Read the model definition and answer for the solid it produces. Units are mm, in the model's axes. A direction names the side the tool comes from. Coordinates: 2 decimals unless noted, no trailing zeros. Loops run counter-clockwise (first coordinate to the right, second up) from the corner with the lowest first, then second, coordinate; pieces in that order, holes last. Notation, with made-up numbers: (14.25, 39.5) - (35.25, 39.5) arc R30 ccw to (35.25, 62.5) - close; hole circle Ø10 at (86.5, 53). An arc over 180 degrees is marked (long way). Use one line per item in the form item = value. Start each with the question number.
1) A cutting plane is placed at A-A (y = 368.3). Give the vertices of the cut face in (x, z) (3 decimals), and give its area (3 significant figures).
2) A cutting plane is placed at B-B (z = -4.5). Give the vertices of the cut face in (x, y) (3 decimals), and give its area (3 significant figures).
3) Which of the six approach directions +Z, -Z, +X, -X, +Y, -Y give full straight-line access (tool end or side, diameter ignored) to faces 1 (the face through (-9.525, 363, 0)), 2 (the face through (-0.279, 730.244, -11.135))?
4) The mould has two halves that part along Y. Classify faces 3 (the face through (-0.279, 730.244, 11.09)), 4 (the face through (9.525, 363, 0)), 5 (the face through (-11, 0, 0)): released by +Y, released by -Y, zero draft, split by the parting line, or undercut.
5) A cutting plane is placed at C-C (y = 555.5). Give the vertices of the cut face in (x, z) (3 decimals).
6) Consider line 1 (Y direction, x = 0, z = -10.25); line 2 (Z direction, x = 3.75, y = 134) (3 decimals); line 3 (X direction, y = 12.7, z = -11.3). Determine where each line is inside the solid, lowest interval first.
7) This flat-tipped pin is pushed along its axis until it touches: P1, Ø14.5, axis at x = 0, y = 368.3, coming from the +Z side. Where does it stop, or does it pass through?
Autodesk Inventor part; units mm, degrees
ref_plane "YZ Plane" through (0, 0, 0) normal (1, 0, 0) x (0, 1, 0)
ref_plane "XZ Plane" through (0, 0, 0) normal (0, 1, 0) x (-1, 0, 0)
ref_plane "XY Plane" through (0, 0, 0) normal (0, 0, 1) x (1, 0, 0)
sketch "Sketch1" plane through (0, 0, 0) normal (0, 1, 0) x (-1, 0, 0)
  line L0 (12.7, 12.7) -> (-12.7, 12.7)
  line L1 (-12.7, 12.7) -> (-12.7, -12.7)
  line L2 (-12.7, -12.7) -> (12.7, -12.7)
  line L3 (12.7, -12.7) -> (12.7, 12.7)
  line L4 (-9.525, 9.525) -> (9.525, 9.525)
  line L5 (9.525, 9.525) -> (9.525, -9.525)
  line L6 (9.525, -9.525) -> (-9.525, -9.525)
  line L7 (-9.525, -9.525) -> (-9.525, 9.525)
  point P0 (0, 0)
  point P1 (12.7, 0)
  point P2 (0, -12.7)
  dimension "d0" = 25.4
  dimension "d1" = 25.4
  dimension "d2" = 3.175
extrude "Extrusion1" add sketch "Sketch1" along normal blind 736.6
sketch "Sketch2" plane through (-12.7, 0, 12.7) normal (0, 0, 1) x (1, 0, 0)
  line L0 (0, 736.6) -> (25.4, 736.6)
  line L1 (0, 0) -> (25.4, 0)
  point P0 (12.7, 0)
  point P1 (12.7, 12.7)
  point P2 (12.7, 723.9)
  point P3 (12.7, 368.3)
  dimension "d5" = 12.7
  dimension "d6" = 12.7
  dimension "d7" = 368.3
hole "Hole1" at (0, 12.7, 12.7) at (0, 723.9, 12.7) at (0, 368.3, 12.7) direction (0, 0, -1) diameter 12.7 end through all
sketch "Sketch3" plane through (-12.7, 0, 12.7) normal (0, 0, 1) x (1, 0, 0)
  line L0 (21.6869, 114.0639) -> (21.6869, 96.9638) construction
  line L1 (21.6869, 96.9638) -> (5.8083, 96.9638) construction
  line L2 (5.8083, 96.9638) -> (5.8083, 114.0639) construction
  line L3 (5.8083, 114.0639) -> (21.6869, 114.0639) construction
  point P0 (12.7, 0)
sketch "Sketch4" plane through (12.7, 0, -12.7) normal (0, 0, -1) x (-1, 0, 0)
  circle A0 centre (12.7, 635.3302) radius 3.175
  line L0 (0, 736.6) -> (25.4, 736.6)
  point P0 (12.7, 0)
  dimension "d15" = 101.2698
  dimension "d16" = 6.35
extrude "Extrusion2" cut sketch "Sketch4" against normal through all
equation "\"d0\" = Tube_size"
equation "\"d1\" = Tube_size"
equation "\"d2\" = Wall_Thickness"
equation "\"d3\" = Bar3_1_Length"
equation "\"d8\" = Pin_Size"
equation "\"Bar1_1_Length\" = 736.6"
equation "\"Tube_size_1\" = 25.4"
equation "\"Wall_Thickness_1\" = 3.175"
equation "\"Lower_Pivit_Offset_FromEdge\" = 12.7"
equation "\"Uper_Pivit_Offset_FromEdge\" = 12.7"
equation "\"Bar1_1_Center_Pivit_Offset_FromEdge\" = 368.3"
equation "\"Bar1_2_Length\" = 736.6"
equation "\"Bar2_1_Length\" = 736.6"
equation "\"Bar2_2_Length\" = 736.6"
equation "\"Bar3_1_Length\" = 736.6"
equation "\"Bar3_2_Length\" = 736.6"
equation "\"Tube_size\" = 25.4"
equation "\"Wall_Thickness\" = 3.175"
equation "\"Bar1_2_Center_Pivit_Offset_FromEdge\" = 368.3"
equation "\"Bar2_1_Center_Pivit_Offset_FromEdge\" = 368.3"
equation "\"Bar2_2_Center_Pivit_Offset_FromEdge\" = 368.3"
equation "\"Bar3_1_Center_Pivit_Offset_FromEdge\" = 368.3"
equation "\"Bar4_2_Center_Pivit_Offset_FromEdge\" = 355.6"
equation "\"Pin_Size\" = 12.7"
equation "\"Bar3_2_Center_Pivit_Offset_FromEdge\" = 368.3"
properties part number "2018 Bar3_1"
Found:
q1.outline = (-12.7, -12.7) - (-6.35, -12.7) - (-6.35, -9.525) - (-9.525, -9.525) - (-9.525, 9.525) - (-6.35, 9.525) - (-6.35, 12.7) - (-12.7, 12.7) - close; (6.35, -12.7) - (12.7, -12.7) - (12.7, 12.7) - (6.35, 12.7) - (6.35, 9.525) - (9.525, 9.525) - (9.525, -9.525) - (6.35, -9.525) - close
q1.area = 202 mm^2
q2.outline = (-12.7, 0) - (-9.525, 0) - (-9.525, 736.6) - (-12.7, 736.6) - close; (9.525, 0) - (12.7, 0) - (12.7, 736.6) - (9.525, 736.6) - close
q2.area = 4,680 mm^2
q3.face_1 = +Y, -Y
q3.face_2 = +Z, -Z
q4.face_3 = undercut
q4.face_4 = zero draft
q4.face_5 = released by -Y
q5.outline = (-12.7, -12.7) - (12.7, -12.7) - (12.7, 12.7) - (-12.7, 12.7) - close; hole (-9.525, -9.525) - (9.525, -9.525) - (9.525, 9.525) - (-9.525, 9.525) - close
q6.line_1 = 0 to 6.35, 19.05 to 361.95, 374.65 to 632.16, 638.51 to 717.55, 730.25 to 736.6
q6.line_2 = -12.7 to -9.525, 9.525 to 12.7
q6.line_3 = -12.7 to -6.35, 6.35 to 12.7
q7.P1 = 12.7
